Geometry check sheet. Reference: the model listing, model coordinates, mm. Coordinates: 2 decimals unless noted, no trailing zeros. Write each loop counter-clockwise with the first axis right and the second up, starting at its lowest first coordinate (ties: lowest second). Pieces come first, ordered by that corner, then holes. Notation, with made-up numbers: (8.5, 45) -> (66.5, 45) arc R32 ccw to (66.5, 73) -> close; hole circle Ø8 at (61.5, 12.5). An arc over 180 degrees is marked (long way). Use a Markdown table: item, result.
```python
from build123d import *

# Parameters (mm, degrees)
BOSS_EXTRUDE1_DEPTH                               = 50
CSK_FOR_4_FLAT_HEAD_MACHINE_SCREW_100_D           = 3.2639
CSK_FOR_4_FLAT_HEAD_MACHINE_SCREW_100_CSINK_D     = 5.715
CSK_FOR_4_FLAT_HEAD_MACHINE_SCREW_100_CSINK_ANGLE = 100
CSK_FOR_4_FLAT_HEAD_MACHINE_SCREW_2_D             = 3.2639
CSK_FOR_4_FLAT_HEAD_MACHINE_SCREW_2_CSINK_D       = 5.715
CSK_FOR_4_FLAT_HEAD_MACHINE_SCREW_2_CSINK_ANGLE   = 100
FILLET1_R                                         = 1
F_2_CLEARANCE_HOLE1_AT_2_COUNT                    = 2
F_2_CLEARANCE_HOLE1_AT_2_PITCH                    = 4.8
CUT_EXTRUDE1_DEPTH                                = 25


with BuildPart() as part:
    # Sketch2 → Boss-Extrude1 (new, symmetric)
    with BuildSketch(Plane.XY):
        with BuildLine():
            Line((-9.525, 0), (9.525, 0))
            Line((9.525, 0), (9.525, 19.05))
            Line((9.525, 19.05), (8.73125, 19.05))
            ThreePointArc((8.73125, 19.05), (8.169983992, 18.817516008), (7.9375, 18.25625))
            Line((7.9375, 18.25625), (7.9375, 2.38125))
            ThreePointArc((7.9375, 2.38125), (7.705016008, 1.819983992), (7.14375, 1.5875))
            Line((7.14375, 1.5875), (-8.73125, 1.5875))
            ThreePointArc((-8.73125, 1.5875), (-9.292516008, 1.355016008), (-9.525, 0.79375))
            Line((-9.525, 0.79375), (-9.525, 0))
        make_face()
    extrude(amount=BOSS_EXTRUDE1_DEPTH, both=True)

    # CSK for _4 Flat Head Machine Screw _100 (through all)
    with Locations(Plane(origin=(0, 0, 0), x_dir=(-1, 0, 0), z_dir=(0, -1, 0))):
        with Locations((4.0625, -46), (4.0625, 46)):
            CounterSinkHole(CSK_FOR_4_FLAT_HEAD_MACHINE_SCREW_100_D / 2, CSK_FOR_4_FLAT_HEAD_MACHINE_SCREW_100_CSINK_D / 2, counter_sink_angle=CSK_FOR_4_FLAT_HEAD_MACHINE_SCREW_100_CSINK_ANGLE)

    # CSK for _4 Flat Head Machine Screw _ 2 (through all)
    with Locations(Plane(origin=(9.525, 0, 0), x_dir=(0, 0, -1), z_dir=(1, 0, 0))):
        with Locations((-46, 9.25), (46, 8.34)):
            CounterSinkHole(CSK_FOR_4_FLAT_HEAD_MACHINE_SCREW_2_D / 2, CSK_FOR_4_FLAT_HEAD_MACHINE_SCREW_2_CSINK_D / 2, counter_sink_angle=CSK_FOR_4_FLAT_HEAD_MACHINE_SCREW_2_CSINK_ANGLE)

    # Fillet1
    fillet1_edges = [part.edges().sort_by_distance(p)[0] for p in [
        (9.525, 0, 0),
    ]]
    fillet(fillet1_edges, radius=FILLET1_R)

    # Sketch30 → #2 Clearance Hole1 (revolve, cut)
    with BuildSketch(Plane(origin=(3.49375, 1.5875, 29.88), x_dir=(0, 0, 1), z_dir=(1, 0, 0))):
        Polygon((0, 0), (0, 1.5875), (2.0574, 1.5875), (1.2192, 0.623261201), (1.2192, 0), align=None)
    f_2_clearance_hole1 = revolve(axis=Axis((3.49375, 7.9375, 29.88), (0, -1, 0)), mode=Mode.SUBTRACT)

    # #2 Clearance Hole1 at 2: #2 Clearance Hole1 ×2
    with Locations(*[(-i * F_2_CLEARANCE_HOLE1_AT_2_PITCH, 0, 0) for i in range(1, F_2_CLEARANCE_HOLE1_AT_2_COUNT)]):
        add(f_2_clearance_hole1, mode=Mode.SUBTRACT)

    # Sketch43 → Cut-Extrude1 (cut)
    with BuildSketch(Plane(origin=(0, 0, -50), x_dir=(-1, 0, 0), z_dir=(0, 0, -1))):
        Polygon((-7.9375, 6.5875), (-7.9375, 1.5875), (-2.9375, 1.5875), align=None)
    cut_extrude1 = extrude(amount=-CUT_EXTRUDE1_DEPTH, mode=Mode.SUBTRACT)

    # Mirror1: Cut-Extrude1 across plane
    add(cut_extrude1.mirror(Plane(origin=(0, 0, 0), x_dir=(1, 0, 0), z_dir=(0, 0, -1))), mode=Mode.SUBTRACT)


solid = part.part
```
Item 1: Thickness scan on L1, parallel to Y at x = 6.25, z = -30.5; L2, parallel to X at y = 15, z = -37 (1 decimal); L3, parallel to Y at x = 8.4, z = -46. Record the ranges inside material, lowest first. Write a range as [from, to].
Answer block:
| item | result |
|---|---|
| L1 | y = [0, 1.59] |
| L2 | x = [7.9, 9.5] |
| L3 | y = [0, 6.71], [9.97, 18.98] |
Item 2: Depth check by flat-ended pin: P1, Ø5, axis at y = 8.34, z = -46, coming from the -X side; P2, Ø3, axis at y = 9.25, z = 46, coming from the +X side; P3, Ø2, axis at x = 1, z = -6.5, coming from the +Y side; P4, Ø4, axis at x = -4.06, z = -46, coming from the -Y side. Enter the tip coordinate at first touch or a pass-through.
Answer block:
| item | result |
|---|---|
| P1 | stops at x = 7.94 |
| P2 | passes through |
| P3 | stops at y = 1.59 |
| P4 | stops at y = 0.72 |
Item 3: Mould release check, pull along Y, two halves, no side actions. Record for faces 1 (the flat face through (-1, 0, 1)), 2 (the cylindrical face through (8.213, 9.443, -47.203)), 3 (the cylindrical face through (-3.19, 1.31, -47.38)): +Y half, -Y half, draft (parallel to the pull), parting line (faces both ways), or undercut.
Answer block:
| item | result |
|---|---|
| face 1 | -Y half |
| face 2 | undercut |
| face 3 | draft |
Item 4: Section check C-C on y = 17.25. Record the boundary of the cut face in (x, z) (1 decimal).
Answer block:
| item | result |
|---|---|
| outline | (7.9, -50) -> (9.5, -50) -> (9.5, 50) -> (7.9, 50) -> close |
Item 5: Section check A-A on z = -46. Count the separate pieces of the cut face and the enclosed holes in it, then the cut area to 3 significant figures.
Answer block:
| item | result |
|---|---|
| separate pieces | 3 |
| enclosed holes | 0 |
| area | 44.6 mm^2 |
